Source: CAD feature listing. Evaluate the final solid. Frame: model axes, mm. Round coordinates to 2 decimals unless told otherwise and drop trailing zeros. Write each loop counter-clockwise with the first axis right and the second up, starting at its lowest first coordinate (ties: lowest second). Pieces come first, ordered by that corner, then holes. Notation, with made-up numbers: M 12,-2.75 L 26,-2.75 A11 cw 26,12.25 Z; hole C -13,25.5 d11. An arc over 180 degrees is marked long. Use a Markdown table: item, result.
Autodesk Inventor part; units mm, degrees
ref_plane "YZ Plane" through (0, 0, 0) normal (1, 0, 0) x (0, 1, 0)
ref_plane "XZ Plane" through (0, 0, 0) normal (0, 1, 0) x (-1, 0, 0)
ref_plane "XY Plane" through (0, 0, 0) normal (0, 0, 1) x (1, 0, 0)
sketch "Esquisse1" plane through (0, 0, 0) normal (0, 1, 0) x (-1, 0, 0)
  line L0 (16.0248, 37.2671) -> (-23.9752, 37.2671)
  line L1 (-23.9752, 37.2671) -> (-23.9752, -42.7329)
  line L2 (-23.9752, -42.7329) -> (16.0248, -42.7329)
  line L3 (16.0248, -42.7329) -> (16.0248, 37.2671)
  point P0 (0, 0)
  dimension "d0" = 80
  dimension "d1" = 40
extrude "Extrusion1" add sketch "Esquisse1" along normal blind 5
sketch "Esquisse2" plane through (0, 0, 0) normal (0, -1, 0) x (1, 0, 0)
  point P0 (0, 0)
sketch "Esquisse3" plane through (0, 0, 0) normal (0, -1, 0) x (1, 0, 0)
  arc A0 (-0.1148, 34.3792) -> (0.3059, 34.1091) centre (-0.7034, 32.9995) ccw
  circle A1 centre (1.7075, 21.9456) radius 1.5
  circle A2 centre (-9.3463, 19.5347) radius 1.5
  circle A3 centre (-11.7572, 30.5885) radius 1.25
  circle A4 centre (-5.0248, 26.2671) radius 4
  circle A5 centre (-0.7034, 32.9995) radius 1.5
  circle A6 centre (-11.7572, 30.5885) radius 1.5
  point P0 (0, 0)
  dimension "d6" = 3
extrude "Extrusion2" cut sketch "Esquisse3" against normal through all contours A5 A0 | A1 | A2 | A3 | A4 | A6
fillet "Congé1" radius 25 1 edges at (23.9752, 2.5, 37.2671)
fillet "Congé2" radius 5 1 edges at (23.9752, 2.5, -42.7329)
fillet "Congé3" radius 5 1 edges at (-16.0248, 2.5, -42.7329)
fillet "Congé4" radius 5 1 edges at (-16.0248, 2.5, 37.2671)
properties part number "trappe"
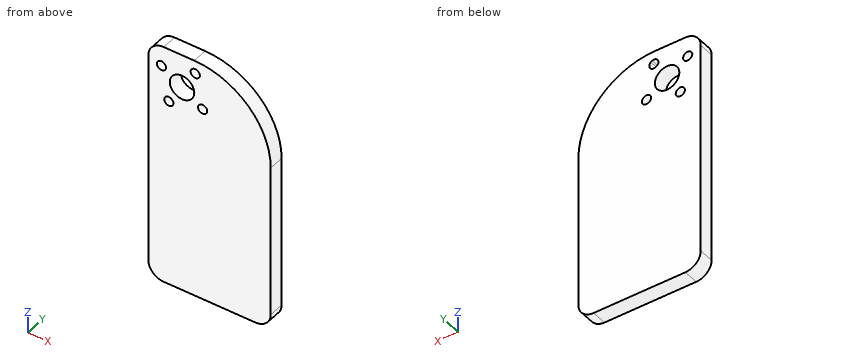
Q1. First-contact query: pin 1 Ø2.5 at (x, z) = (1.71, 21.95) entering from +Y; pin 2 Ø3.5 at (x, z) = (-9.35, 19.53) entering from +Y. Flat tips, straight axial feed; report the tip coordinate or a pass-through.
Results are:
| item | result |
|---|---|
| pin 1 | through |
| pin 2 | y = 5 |
Q2. Line query: L1, parallel to X at y = 3.1, z = -38; L2, parallel to Z at x = -6.5, y = 3.7; L3, parallel to Z at x = 0, y = 4.1. Output: solid intervals per line, ascending.
Results are:
| item | result |
|---|---|
| L1 | -16.02 to 23.97 |
| L2 | -42.73 to 22.55, 29.99 to 37.27 |
| L3 | -42.73 to 31.67, 34.32 to 37.25 |
Q3. Section C-C on x = 14.5. Return loops of the section in (y, z).
Results are:
| item | result |
|---|---|
| outline | M 0,-42.73 L 5,-42.73 L 5,31.86 L 0,31.86 Z |
Q4. Section B-B on y = 1.35. Return loops of the section in (x, z), plus the area to 3 significant figures.
Results are:
| item | result |
|---|---|
| outline | M -16.02,-37.73 A5 ccw -11.02,-42.73 L 18.98,-42.73 A5 ccw 23.98,-37.73 L 23.98,12.27 A25 ccw -1.02,37.27 L -11.02,37.27 A5 ccw -16.02,32.27 Z; hole C -11.76,30.59 d3; hole C -9.35,19.53 d3; hole C -5.02,26.27 d8; hole M -0.11,34.38 A1.5 ccw long 0.31,34.11 A1.5 ccw Z; hole C 1.71,21.95 d3 |
| area | 2,970 mm^2 |
Q5. Section A-A on x = -4. Return loops of the section in (y, z).
Results are:
| item | result |
|---|---|
| outline | M 0,-42.73 L 5,-42.73 L 5,22.4 L 0,22.4 Z; M 0,30.13 L 5,30.13 L 5,37.27 L 0,37.27 Z |
